The model under review builds one solid part; all positions refer to its coordinate system, in mm. Face numbers are marked on the shaded views. A direction names the side the tool comes from. Give positions to 0.01 mm unless a question says otherwise; leave off trailing zeros. Loops run counter-clockwise (first coordinate to the right, second up) from the corner with the lowest first, then second, coordinate; pieces in that order, holes last. Notation, with made-up numbers: (70.25, -31.5) - (126.25, -31.5) arc R19 ccw to (126.25, -2.5) - close; hole circle Ø9 at (16.5, 56). An arc over 180 degrees is marked (long way). Answer as a JSON object with one key per item and string values.
from build123d import *

# Parameters (mm, degrees)
SKETCH1_W           = 64.1
SKETCH1_H           = 75
BOSS_EXTRUDE1_DEPTH = 3
SKETCH1_4_W         = 3
SKETCH1_4_H         = 75
BOSS_EXTRUDE2_DEPTH = 58
SKETCH2_R           = 22.5
CUT_EXTRUDE1_DEPTH  = 10
FILLET2_R           = 16
BOSS_EXTRUDE3_START = 55
BOSS_EXTRUDE3_DEPTH = 55
SKETCH5_R           = 14
SKETCH5_R_2         = 1.6
CUT_EXTRUDE2_DEPTH  = 129.681816897
SKETCH7_W           = 43.224612372
SKETCH7_H           = 24
CUT_EXTRUDE3_DEPTH  = 10
SKETCH5_5_W         = 23.859751581
SKETCH5_5_H         = 20.349819761
CUT_EXTRUDE5_DEPTH  = 74
BOSS_EXTRUDE4_DEPTH = 7
SKETCH9_4_W         = 15
SKETCH9_4_H         = 3
BOSS_EXTRUDE5_DEPTH = 16


with BuildPart() as part:
    # Sketch1 → Boss-Extrude1 (new body)
    with BuildSketch(Plane(origin=(0, 0, 0), x_dir=(1, 0, 0), z_dir=(0, 1, 0))):
        Polygon((64.1, 75), (67.1, 75), (67.1, 91), (-3, 91), (-3, 75), (0, 75), align=None)
        with Locations((32.05, 37.5)):
            Rectangle(SKETCH1_W, SKETCH1_H)
        Polygon((67.1, 0), (67.1, -16), (-3, -16), (-3, 0), (0, 0), (64.1, 0), align=None)
    extrude(amount=BOSS_EXTRUDE1_DEPTH)

    # Sketch1<4> → Boss-Extrude2 (add)
    with BuildSketch(Plane(origin=(0, 0, 0), x_dir=(1, 0, 0), z_dir=(0, 1, 0))):
        with Locations((65.6, 37.5)):
            Rectangle(SKETCH1_4_W, SKETCH1_4_H)
        with Locations((-1.5, 37.5)):
            Rectangle(SKETCH1_4_W, SKETCH1_4_H)
    extrude(amount=BOSS_EXTRUDE2_DEPTH)

    # Sketch2 → Cut-Extrude1 (cut)
    with BuildSketch(Plane.XZ):
        with Locations(Location((32.05, -51.354505882, 0), (0, 0, 270))):
            Circle(SKETCH2_R)
    extrude(amount=-CUT_EXTRUDE1_DEPTH, mode=Mode.SUBTRACT)

    # Fillet2
    fillet2_edges = [part.edges().sort_by_distance(p)[0] for p in [
        (-3, 1.5, -91),
        (67.1, 1.5, -91),
        (67.1, 1.5, 16),
        (-3, 1.5, 16),
    ]]
    fillet(fillet2_edges, radius=FILLET2_R)

    # Sketch6 → Boss-Extrude3 (add)
    with BuildSketch(Plane(origin=(0, 3, 0), x_dir=(1, 0, 0), z_dir=(0, 1, 0)).offset(BOSS_EXTRUDE3_START)):
        with BuildLine():
            Line((3, 83.306623863), (3, 87.489995997))
            ThreePointArc((3, 87.489995997), (-1.422205102, 81.92820323), (-3, 75))
            Line((-3, 75), (0, 75))
            ThreePointArc((0, 75), (0.772980739, 79.415880433), (3, 83.306623863))
        make_face()
        with BuildLine():
            Line((61.1, 87.489995997), (61.1, 83.306623863))
            ThreePointArc((61.1, 83.306623863), (63.327019261, 79.415880433), (64.1, 75))
            Line((64.1, 75), (67.1, 75))
            ThreePointArc((67.1, 75), (65.522205102, 81.92820323), (61.1, 87.489995997))
        make_face()
        with BuildLine():
            Line((64.1, 0), (67.1, 0))
            ThreePointArc((67.1, 0), (62.413708499, -11.313708499), (51.1, -16))
            Line((51.1, -16), (13, -16))
            ThreePointArc((13, -16), (1.686291501, -11.313708499), (-3, 0))
            Line((-3, 0), (0, 0))
            ThreePointArc((0, 0), (3.807611845, -9.192388155), (13, -13))
            Line((13, -13), (51.1, -13))
            ThreePointArc((51.1, -13), (60.292388155, -9.192388155), (64.1, 0))
        make_face()
    extrude(amount=-BOSS_EXTRUDE3_DEPTH)

    # Sketch5 → Cut-Extrude2 (cut, through all)
    with BuildSketch(Plane.ZY.offset(3)):
        with Locations((-57.920720454, 30.91264254)):
            Circle(SKETCH5_R)
        with Locations((-69.920720454, 42.91264254)):
            Circle(SKETCH5_R_2)
        with Locations((-69.920720454, 18.91264254)):
            Circle(SKETCH5_R_2)
        with Locations((-45.920720454, 18.91264254)):
            Circle(SKETCH5_R_2)
        with Locations((-45.920720454, 42.91264254)):
            Circle(SKETCH5_R_2)
    extrude(amount=-CUT_EXTRUDE2_DEPTH, mode=Mode.SUBTRACT)

    # Sketch7 → Cut-Extrude3 (cut)
    with BuildSketch(Plane(origin=(67.1, 0, 0), x_dir=(0, 0, -1), z_dir=(1, 0, 0))):
        with Locations((65.877689811, 46)):
            Rectangle(SKETCH7_W, SKETCH7_H)
    extrude(amount=-CUT_EXTRUDE3_DEPTH, mode=Mode.SUBTRACT)

    # Sketch5<5> → Cut-Extrude5 (cut)
    with BuildSketch(Plane.ZY.offset(3)):
        Polygon((0, 58), (0, 42.024482082), (23.859751581, 42.024482082), (23.859751581, 64.276966148), (0, 64.276966148), align=None)
        with Locations((11.929875791, 31.849572202)):
            Rectangle(SKETCH5_5_W, SKETCH5_5_H)
        Polygon((0, 21.674662321), (0, 42.024482082), (-10.174909881, 31.849572202), align=None)
    extrude(amount=-CUT_EXTRUDE5_DEPTH, mode=Mode.SUBTRACT)

    # Sketch9 → Boss-Extrude4 (add)
    with BuildSketch(Plane.ZY.offset(-64.1)):
        Polygon((0, 58), (-44.265383625, 58), (-44.265383625, 50), (-29.265383625, 50), (-14.265383625, 50), (0, 50), align=None)
    extrude(amount=BOSS_EXTRUDE4_DEPTH)

    # Sketch9<4> → Boss-Extrude5 (add)
    with BuildSketch(Plane.ZY.offset(-64.1)):
        with Locations((-21.765383625, 48.5)):
            Rectangle(SKETCH9_4_W, SKETCH9_4_H)
    extrude(amount=BOSS_EXTRUDE5_DEPTH)


solid = part.part
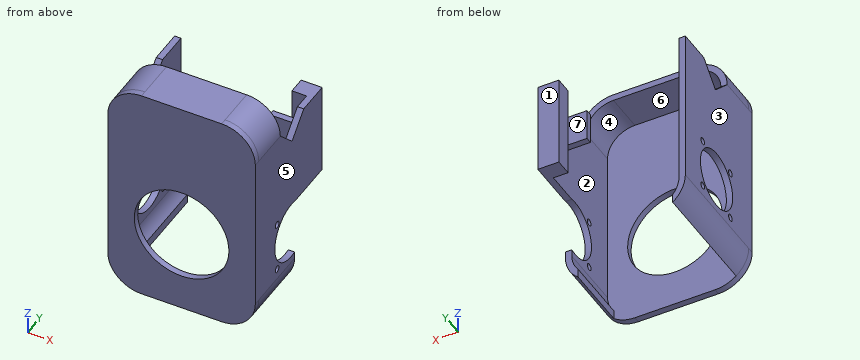
Q1. Consider section C-C, the plane x = 58.5. State the section outline as (y, z) points, plus the area to 3 significant figures.
Results:
{"outline": "(0, -89.19) - (3, -89.19) - (3, 10.69) - (21.67, 10.69) - (21.67, 14.19) - (0, 14.19) - close; (47, -29.27) - (50, -29.27) - (50, -44.27) - (58, -44.27) - (58, 0) - (50, 0) - (50, -14.27) - (47, -14.27) - close", "area": "775 mm^2"}
Q2. Clearance check with flat-ended pins moving along their axes: pin 1 Ø5 at (x, y) = (63.5, 46.5) entering from +Z; pin 2 Ø4.5 at (y, z) = (28, -85) entering from +X; pin 3 Ø5.5 at (x, y) = (32, 12.5) entering from -Z; pin 4 Ø10 at (x, y) = (55.5, 38.5) entering from +Z. State where each tip first meets the part, or that it passes through.
Results:
{"pin 1": "stops at z = 0", "pin 2": "stops at x = 65.1", "pin 3": "stops at z = 13", "pin 4": "passes through"}
Q3. Consider section B-B, the plane z = -53.5. State the section outline as (x, y) points, plus the area to 3 significant figures.
Results:
{"outline": "(-3, 0) - (9.65, 0) - (9.65, 3) - (0, 3) - (0, 17.63) - (-3, 17.63) - close; (-3, 44.2) - (0, 44.2) - (0, 58) - (-3, 58) - close; (54.45, 0) - (67.1, 0) - (67.1, 17.63) - (64.1, 17.63) - (64.1, 3) - (54.45, 3) - close", "area": "205 mm^2"}
Q4. To check wall thickness, follow probe 1 along X at (y, z) = (24, -31); probe 2 along Y at (x, z) = (49, -80.5); probe 3 along Z at (x, y) = (12.5, 12). State the ranges of each line that lie inside material, in increasing order. Write a range as [from, to].
Results:
{"probe 1": "x = [-3, 0], [64.1, 67.1]", "probe 2": "y = [0, 3]", "probe 3": "z = [12.99, 15.99]"}
Q5. Consider section D-D, the plane z = -81. State the section outline as (x, y) points.
Results:
{"outline": "(-1.83, 0) - (65.93, 0) - (65.93, 34) - (62.63, 34) - (62.63, 3) - (1.47, 3) - (1.47, 58) - (-1.83, 58) - close"}
Q6. Consider section A-A, the plane x = 32.05. State the section outline as (y, z) points, plus the area to 3 significant figures.
Results:
{"outline": "(0, -91) - (3, -91) - (3, -73.85) - (0, -73.85) - close; (0, -28.85) - (3, -28.85) - (3, 13) - (21.67, 13) - (21.67, 16) - (0, 16) - close", "area": "242 mm^2"}
Q7. For the marked faces 4, 5, 6 and 7, list the 3-axis set-ups (+Z, -Z, +X, -X, +Y, -Y) from which the entire face can be reached by the end or side of a thin tool; tool diameter is ignored.
Results:
{"face 4": "+Y", "face 5": "+Z, -Z, +X, +Y, -Y", "face 6": "-Z, +Y", "face 7": "+Z, -Z, +Y"}
Q8. The part is to be moulded in two halves that separate along Y. For the marked faces 1, 2 and 3, say which applies: +Y half, -Y half, draft (parallel to the pull), parting line (faces both ways), or undercut.
Results:
{"face 1": "+Y half", "face 2": "undercut", "face 3": "draft"}
